```python
from build123d import *

# Parameters (mm, degrees)
SKETCH1_W           = 27
SKETCH1_H           = 72.2
SKETCH1_R           = 11
SKETCH1_R_2         = 3.25
SKETCH1_R_3         = 5.75
SKETCH1_R_4         = 1.5
BOSS_EXTRUDE1_DEPTH = 50
BOSS_EXTRUDE3_DEPTH = 72.2
CUT_EXTRUDE2_DEPTH  = 35
SKETCH1_3_R         = 11
SKETCH1_3_R_2       = 5.75
SKETCH1_3_R_3       = 1.5
CUT_EXTRUDE1_DEPTH  = 47
SKETCH3_R           = 22.5
SKETCH3_R_2         = 10
SKETCH3_R_3         = 2
CUT_EXTRUDE3_DEPTH  = 37.2
SKETCH3_6_R         = 22.5
SKETCH3_6_R_2       = 2
SKETCH3_6_R_3       = 10
BOSS_EXTRUDE4_DEPTH = 5
FILLET1_R           = 10


# Read off the part's stored shape, not the designer's step: Cut-Extrude2
with BuildPart() as part:
    # Sketch1 → Boss-Extrude1 (new body)
    # profile 1 of 2: a face of its own
    with BuildSketch(Plane(origin=(0, 0, 0), x_dir=(0, 0, -1), z_dir=(1, 0, 0))):
        Rectangle(SKETCH1_W, SKETCH1_H)
        Circle(SKETCH1_R, mode=Mode.SUBTRACT)
        with Locations((0, -28.75)):
            Circle(SKETCH1_R_2, mode=Mode.SUBTRACT)
        with Locations((0, 28.75)):
            Circle(SKETCH1_R_2, mode=Mode.SUBTRACT)
    # profile 2 of 2: a face of its own
    with BuildSketch(Plane(origin=(0, 0, 0), x_dir=(0, 0, -1), z_dir=(1, 0, 0))):
        Circle(SKETCH1_R)
        Circle(SKETCH1_R_3, mode=Mode.SUBTRACT)
        with Locations((-5.656854249, 5.656854249)):
            Circle(SKETCH1_R_4, mode=Mode.SUBTRACT)
        with Locations((5.656854249, 5.656854249)):
            Circle(SKETCH1_R_4, mode=Mode.SUBTRACT)
        with Locations((5.656854249, -5.656854249)):
            Circle(SKETCH1_R_4, mode=Mode.SUBTRACT)
        with Locations((-5.656854249, -5.656854249)):
            Circle(SKETCH1_R_4, mode=Mode.SUBTRACT)
    extrude(amount=BOSS_EXTRUDE1_DEPTH)

    # Sketch2 → Boss-Extrude3 (add)
    with BuildSketch(Plane(origin=(0, -36.1, 0), x_dir=(1, 0, 0), z_dir=(0, 1, 0))):
        with BuildLine():
            Line((0, 13.5), (25, 13.5))
            ThreePointArc((25, 13.5), (7.32233047, 20.82233047), (0, 38.5))
            Line((0, 38.5), (0, 13.5))
        make_face()
        with BuildLine():
            ThreePointArc((25, 13.5), (42.67766953, 20.82233047), (50, 38.5))
            Line((50, 38.5), (0, 38.5))
            ThreePointArc((0, 38.5), (7.32233047, 20.82233047), (25, 13.5))
        make_face()
        with BuildLine():
            Line((25, 13.5), (50, 13.5))
            Line((50, 13.5), (50, 38.5))
            ThreePointArc((50, 38.5), (42.67766953, 20.82233047), (25, 13.5))
        make_face()
        with BuildLine():
            Line((0, 38.5), (50, 38.5))
            ThreePointArc((50, 38.5), (25, 63.5), (0, 38.5))
        make_face()
    extrude(amount=BOSS_EXTRUDE3_DEPTH)

    # Cut-Extrude2 outline → Cut-Extrude2 (cut)
    with BuildSketch(Plane(origin=(0, -36.1, 0), x_dir=(1, 0, 0), z_dir=(0, 1, 0))):
        with BuildLine():
            Line((0, 13.5), (50, 13.5))
            Line((50, 13.5), (50, 38.5))
            ThreePointArc((50, 38.5), (25, 63.5), (0, 38.5))
            Line((0, 38.5), (0, 13.5))
        make_face()
    extrude(amount=CUT_EXTRUDE2_DEPTH, mode=Mode.SUBTRACT)

    # Sketch1<3> → Cut-Extrude1 (cut)
    with BuildSketch(Plane(origin=(0, 0, 0), x_dir=(0, 0, -1), z_dir=(1, 0, 0))):
        Circle(SKETCH1_3_R)
        Circle(SKETCH1_3_R_2, mode=Mode.SUBTRACT)
        with Locations((-5.656854249, 5.656854249)):
            Circle(SKETCH1_3_R_3, mode=Mode.SUBTRACT)
        with Locations((5.656854249, 5.656854249)):
            Circle(SKETCH1_3_R_3, mode=Mode.SUBTRACT)
        with Locations((5.656854249, -5.656854249)):
            Circle(SKETCH1_3_R_3, mode=Mode.SUBTRACT)
        with Locations((-5.656854249, -5.656854249)):
            Circle(SKETCH1_3_R_3, mode=Mode.SUBTRACT)
    extrude(amount=CUT_EXTRUDE1_DEPTH, mode=Mode.SUBTRACT)

    # Sketch3 → Cut-Extrude3 (cut)
    # profile 1 of 6: a face of its own
    with BuildSketch(Plane.XZ.offset(1.1)):
        with Locations(Location((25, -38.5, 0), (0, 0, 270))):
            Circle(SKETCH3_R)
        with Locations((25, -38.5)):
            Circle(SKETCH3_R_2, mode=Mode.SUBTRACT)
        with Locations((15, -48.5)):
            Circle(SKETCH3_R_3, mode=Mode.SUBTRACT)
        with Locations((35, -48.5)):
            Circle(SKETCH3_R_3, mode=Mode.SUBTRACT)
        with Locations((35, -28.5)):
            Circle(SKETCH3_R_3, mode=Mode.SUBTRACT)
        with Locations((15, -28.5)):
            Circle(SKETCH3_R_3, mode=Mode.SUBTRACT)
    # profile 2 of 6: a face of its own
    with BuildSketch(Plane.XZ.offset(1.1)):
        with Locations((25, -38.5)):
            Circle(SKETCH3_R_2)
    # profile 3 of 6: a face of its own
    with BuildSketch(Plane.XZ.offset(1.1)):
        with Locations((35, -28.5)):
            Circle(SKETCH3_R_3)
    # profile 4 of 6: a face of its own
    with BuildSketch(Plane.XZ.offset(1.1)):
        with Locations((15, -28.5)):
            Circle(SKETCH3_R_3)
    # profile 5 of 6: a face of its own
    with BuildSketch(Plane.XZ.offset(1.1)):
        with Locations((15, -48.5)):
            Circle(SKETCH3_R_3)
    # profile 6 of 6: a face of its own
    with BuildSketch(Plane.XZ.offset(1.1)):
        with Locations((35, -48.5)):
            Circle(SKETCH3_R_3)
    extrude(amount=-CUT_EXTRUDE3_DEPTH, mode=Mode.SUBTRACT)

    # Sketch3<6> → Boss-Extrude4 (add)
    with BuildSketch(Plane.XZ.offset(1.1)):
        with Locations(Location((25, -38.5, 0), (0, 0, 270))):
            Circle(SKETCH3_6_R)
        with Locations(Location((15, -28.5, 0), (0, 0, 270))):
            Circle(SKETCH3_6_R_2, mode=Mode.SUBTRACT)
        with Locations(Location((35, -28.5, 0), (0, 0, 270))):
            Circle(SKETCH3_6_R_2, mode=Mode.SUBTRACT)
        with Locations(Location((35, -48.5, 0), (0, 0, 270))):
            Circle(SKETCH3_6_R_2, mode=Mode.SUBTRACT)
        with Locations(Location((15, -48.5, 0), (0, 0, 270))):
            Circle(SKETCH3_6_R_2, mode=Mode.SUBTRACT)
        with Locations(Location((25, -38.5, 0), (0, 0, 270))):
            Circle(SKETCH3_6_R_3, mode=Mode.SUBTRACT)
    extrude(amount=-BOSS_EXTRUDE4_DEPTH)

    # Fillet1
    fillet1_edges = [part.edges().sort_by_distance(p)[0] for p in [
        (25, 36.1, 13.5),
        (25, -36.1, 13.5),
        (25, -36.1, -13.5),
    ]]
    fillet(fillet1_edges, radius=FILLET1_R)


solid = part.part
```
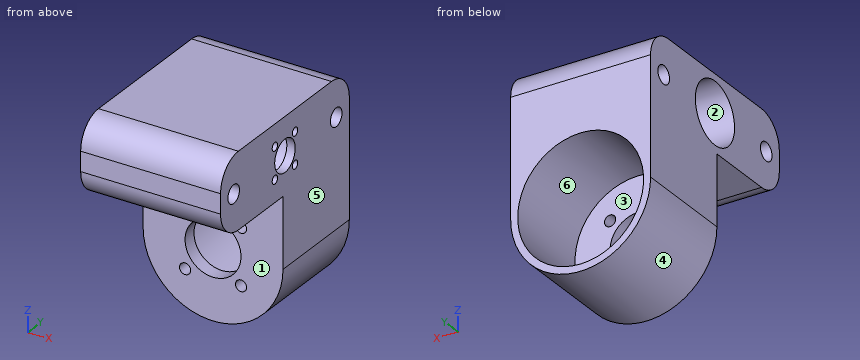
CAD build for the part. Positions are in the model's coordinates, mm. Face numbers are marked on the shaded views. A direction names the side the tool comes from. Round coordinates to 2 decimals unless told otherwise and drop trailing zeros. Write each loop counter-clockwise with the first axis right and the second up, starting at its lowest first coordinate (ties: lowest second). Pieces come first, ordered by that corner, then holes. Notation, with made-up numbers: M 45.5,79.5 L 104.5,79.5 A31 ccw 104.5,106.5 Z; hole C 60,-21.5 d2. An arc over 180 degrees is marked long. One line per question, with ' | ' between items.
1. Cut at B-B on z = 0. Write the cut outline in (x, y), and give its area (3 significant figures).
Working result:
outline: M 0,-36.1 L 50,-36.1 L 50,-32 L 0,-32 Z; M 0,-25.5 L 50,-25.5 L 50,-5.75 L 47,-5.75 L 47,-11 L 0,-11 Z; M 0,11 L 47,11 L 47,5.75 L 50,5.75 L 50,25.5 L 0,25.5 Z; M 0,32 L 50,32 L 50,36.1 L 0,36.1 Z | area: 1,890 mm2
2. Cut at D-D on z = -27.5. Write the cut outline in (x, y), and give its area (3 significant figures).
Working result:
outline: M 0,-1.1 L 13.27,-1.1 L 13.27,3.9 L 5.37,3.9 L 5.37,36.1 L 0,36.1 Z; M 16.73,-1.1 L 33.27,-1.1 L 33.27,3.9 L 16.73,3.9 Z; M 36.73,-1.1 L 50,-1.1 L 50,36.1 L 44.63,36.1 L 44.63,3.9 L 36.73,3.9 Z | area: 561 mm2
3. Probe L1, parallel to Y at x = 29.5, z = 0.5; L2, parallel to Y at x = 12, z = -2; L3, parallel to Z at x = 23, y = 29. List the from-to ranges inside material, lowest first. Write a range as from..to.
Working result:
L1: -36.1..-31.96, -25.54..-10.99, 10.99..25.54, 31.96..36.1 | L2: -36.1..-31.31, -26.19..-10.82, 10.82..26.19, 31.31..36.1 | L3: -63.42..-60.91, -16.09..-3.24, 3.24..13.07
4. Pin check, flat tips, straight feed: pin 1 Ø1.5 at (x, y) = (26.5, -28.5) entering from +Z; pin 2 Ø10 at (x, z) = (5.5, -9) entering from -Y; pin 3 Ø4.5 at (x, z) = (35, -48.5) entering from -Y. Stop position of each tip, or through.
Working result:
pin 1: z = 13.36 | pin 2: y = -36.09 | pin 3: y = -1.1
5. Cut at C-C on y = 28.75. Write the cut outline in (x, z), and give its area (3 significant figures).
Working result:
outline: M 0,-38.5 A25 ccw 50,-38.5 L 50,-3.25 L 0,-3.25 Z; M 0,3.25 L 50,3.25 L 50,13.14 L 0,13.14 Z; hole C 25,-38.5 d45 | area: 1,650 mm2
6. Which spindle directions (+Z, -Z, +X, -X, +Y, -Y) get a long thin tool onto all of the face, cutting with end or side? Do the marked faces 1, 2 and 3. Say none if no direction does.
Working result:
face 1: -Z, +X, -X, -Y | face 2: -X | face 3: +Y
7. Mould opens along X. For the marked faces 4, 5 and 6 say: pulls with the +X half, pulls with the -X half, needs draft (parallel to the pull), parting line crosses it, or undercut.
Working result:
face 4: parting line crosses it | face 5: pulls with the +X half | face 6: undercut
8. Cut at A-A on x = 25. Write the cut outline in (y, z).
Working result:
outline: M -36.1,-3.5 A10 ccw -26.1,-13.5 L -1.1,-13.5 L -1.1,-28.5 L 3.9,-28.5 L 3.9,-16 L 36.1,-16 L 36.1,3.5 A10 ccw 26.1,13.5 L -26.1,13.5 A10 ccw -36.1,3.5 Z; M -1.1,-63.5 L 36.1,-63.5 L 36.1,-61 L 3.9,-61 L 3.9,-48.5 L -1.1,-48.5 Z; hole C -28.75,0 d6.5; hole C 0,0 d22; hole C 28.75,0 d6.5
